Autodesk Inventor part; units mm, degrees
ref_plane "YZ Plane" through (0, 0, 0) normal (1, 0, 0) x (0, 1, 0)
ref_plane "XZ Plane" through (0, 0, 0) normal (0, 1, 0) x (-1, 0, 0)
ref_plane "XY Plane" through (0, 0, 0) normal (0, 0, 1) x (1, 0, 0)
sketch "Sketch1" plane through (0, 0, 0) normal (0, 1, 0) x (-1, 0, 0)
  line L0 (2.286, 0) -> (10.414, 0)
  line L1 (12.7, -2.286) -> (12.7, -10.414)
  line L2 (10.414, -12.7) -> (2.286, -12.7)
  line L3 (0, -10.414) -> (0, -2.286)
  line L4 (8.1534, -4.0386) -> (4.5466, -4.0386)
  line L5 (4.0386, -4.5466) -> (4.0386, -8.1534)
  line L6 (4.5466, -8.6614) -> (8.1534, -8.6614)
  line L7 (8.6614, -8.1534) -> (8.6614, -4.5466)
  line L8 (10.414, 0) -> (12.7, -2.286)
  line L9 (12.7, -10.414) -> (10.414, -12.7)
  line L10 (2.286, -12.7) -> (0, -10.414)
  line L11 (2.286, 0) -> (0, -2.286)
  arc A0 (8.6614, -4.5466) -> (8.1534, -4.0386) centre (8.1534, -4.5466) ccw
  arc A1 (8.1534, -8.6614) -> (8.6614, -8.1534) centre (8.1534, -8.1534) ccw
  arc A2 (4.0386, -8.1534) -> (4.5466, -8.6614) centre (4.5466, -8.1534) ccw
  arc A3 (4.5466, -4.0386) -> (4.0386, -4.5466) centre (4.5466, -4.5466) ccw
  line L12 (8.1534, -4.5466) -> (4.5466, -8.1534) construction
  line L13 (12.7, -10.414) -> (0, -2.286) construction
  point P0 (0, 0)
  point P1 (12.7, -12.7)
  point P2 (12.7, 0)
  point P3 (0, -12.7)
  point P4 (4.0386, -8.6614)
  point P5 (8.6614, -8.6614)
  point P6 (6.35, -6.35)
  dimension "d1" = 12.7
  dimension "d2" = 4.6228
  dimension "d3" = 2.286
  dimension "d4" = 2.286
  dimension "d5" = 2.286
  dimension "d6" = 2.286
  dimension "d7" = 2.286
  dimension "d8" = 2.286
  dimension "d9" = 2.286
  dimension "d10" = 2.286
  dimension "d11" = 0.508
extrude "Body" add sketch "Sketch1" along normal blind 1.1906
sketch "Sketch2" plane through (0, 1.1906, 0) normal (0, 1, 0) x (1, 0, 0)
  arc A0 (-8.1534, 8.6614) -> (-8.6614, 8.1534) centre (-8.1534, 8.1534) ccw construction
  arc A1 (-4.5466, 4.0386) -> (-4.0386, 4.5466) centre (-4.5466, 4.5466) ccw construction
  circle A2 centre (-6.35, 6.35) radius 2.1844
  line L0 (-8.1534, 8.1534) -> (-4.5466, 4.5466) construction
  point P0 (0, 0)
  dimension "d14" = 4.3688
surface extrude "Circle" sketch "Sketch2" against normal up to surface (1.1906 mm away) shown yes curves A2
pattern_of_one "Rectangular Pattern1"
equation "\"d22\" = d19"
Source: CAD feature listing. Evaluate the final solid. Frame: model axes, mm. A direction names the side the tool comes from. Round coordinates to 2 decimals unless told otherwise and drop trailing zeros. Write each loop counter-clockwise with the first axis right and the second up, starting at its lowest first coordinate (ties: lowest second). Pieces come first, ordered by that corner, then holes. Notation, with made-up numbers: M 74,-38 L 97,-38 A27 ccw 97,-14 Z; hole C -20,-6.75 d8. An arc over 180 degrees is marked long. Answer as a JSON object with one key per item and string values. Group by question number.
(1) Reachability of faces 1 (the flat face through (-8.661, 1, -6)), 2 (the flat face through (-11.541, 0.587, -1.127)) from +Z, -Z, +X, -X, +Y, -Y: full face, straight path, thin tool, end or side. Return the list, or none.
(2) Ray query, line 1 (Z direction, x = -6.25, y = 0.75); line 2 (Z direction, x = -11.25, y = 0.75). Return the intervals inside material, ascending. Write a range as [from, to].
(3) Section query C-C on y = 0.35. Output: boundary loops of the cut face in (x, z).
(4) Section query B-B on x = -6. Output: boundary loops of the cut face in (y, z).
(5) Section query A-A on z = -5. Output: boundary loops of the cut face in (x, y), then the cut area to 3 significant figures.
(6) Section query D-D on x = -11.5. Output: boundary loops of the cut face in (y, z).
Computed values:
{
 "1": {"face 1": "+Y, -Y", "face 2": "+Z, -X, +Y, -Y"},
 "2": {"line 1": "[-12.7, -8.66], [-4.04, 0]", "line 2": "[-11.86, -0.84]"},
 "3": {"outline": "M -12.7,-10.41 L -10.41,-12.7 L -2.29,-12.7 L 0,-10.41 L 0,-2.29 L -2.29,0 L -10.41,0 L -12.7,-2.29 Z; hole M -8.66,-8.15 A0.51 ccw -8.15,-8.66 L -4.55,-8.66 A0.51 ccw -4.04,-8.15 L -4.04,-4.55 A0.51 ccw -4.55,-4.04 L -8.15,-4.04 A0.51 ccw -8.66,-4.55 Z"},
 "4": {"outline": "M 0,-12.7 L 1.19,-12.7 L 1.19,-8.66 L 0,-8.66 Z; M 0,-4.04 L 1.19,-4.04 L 1.19,0 L 0,0 Z"},
 "5": {"outline": "M -12.7,0 L -8.66,0 L -8.66,1.19 L -12.7,1.19 Z; M -4.04,0 L 0,0 L 0,1.19 L -4.04,1.19 Z", "area": "9.62 mm^2"},
 "6": {"outline": "M 0,-11.61 L 1.19,-11.61 L 1.19,-1.09 L 0,-1.09 Z"}
}
